Read the model definition and answer for the solid it produces. Units are mm, in the model's axes. A direction names the side the tool comes from. Coordinates: 2 decimals unless noted, no trailing zeros. Write each loop counter-clockwise with the first axis right and the second up, starting at its lowest first coordinate (ties: lowest second). Pieces come first, ordered by that corner, then holes. Notation, with made-up numbers: (-35.75, -10) -> (0.25, -10) arc R30 cw to (0.25, 19) -> close; hole circle Ø11 at (1, 86.25). An arc over 180 degrees is marked (long way). Write item = value, one per line. Start each with the question number.
1) Flat-ended cylindrical pins translate along their axes: pin 1 Ø5 at (x, z) = (10, 192.75) entering from +Y; pin 2 Ø5 at (y, z) = (10, 207) entering from +X. Find the tip coordinate at first contact, or state that the pin passes through.
2) A tool of negligible diameter and unlimited length cuts with its end or side. For faces 1 (the face through (4, 6, 0)), 2 (the face through (10, 5, 173)), from which of +Z, -Z, +X, -X, +Y, -Y can it reach the whole face along a straight path? Write none if from no direction.
3) Section A-A (y = 2.75) is taken. Count the separate pieces of the cut face and the enclosed holes in it, plus the area to 3 significant figures.
4) Find the intervals of material crossed by line 1 along X through (y, z) = (2.5, 342.55); line 2 along X through (y, z) = (12.25, 227), in increasing order. Write a range as from..to.
5) Section B-B (z = 247.5) is taken. Determine the outline of the cut face in (x, y), plus the area to 3 significant figures.
from build123d import *

# Parameters (mm, degrees)
BOSS_EXTRUDE1_DEPTH                  = 350
F_3_2_3_2_DIAMETER_HOLE1_D           = 3.2
LPATTERN2_COUNT                      = 4
LPATTERN2_PITCH                      = 74.9
F_3_2_3_2_DIAMETERHOLEFORAHALFPART_D = 3.2


with BuildPart() as part:
    # Sketch1 → Boss-Extrude1 (new body)
    with BuildSketch(Plane.XY):
        Polygon((0, 0), (0, 15), (5, 15), (5, 5), (15, 5), (15, 0), align=None)
    extrude(amount=BOSS_EXTRUDE1_DEPTH)

    # Ø3.2 (3.2) Diameter Hole1 (through all)
    with Locations(Plane(origin=(0, 0, 0), x_dir=(-1, 0, 0), z_dir=(0, -1, 0))):
        with Locations((-10, -342.55), (-10, -282.55)):
            f_3_2_3_2_diameter_hole1 = Hole(F_3_2_3_2_DIAMETER_HOLE1_D / 2)

    # LPattern2: Ø3.2 (3.2) Diameter Hole1 ×4
    with Locations(*[(0, 0, -i * LPATTERN2_PITCH) for i in range(1, LPATTERN2_COUNT)]):
        add(f_3_2_3_2_diameter_hole1, mode=Mode.SUBTRACT)

    # Ø3.2 (3.2) DiameterHoleForAHalfPart (through all)
    with Locations(Plane(origin=(0, 0, 0), x_dir=(-1, 0, 0), z_dir=(0, -1, 0))):
        with Locations((-10, -42.95), (-10, -12.95)):
            Hole(F_3_2_3_2_DIAMETERHOLEFORAHALFPART_D / 2)


solid = part.part
Answer key:
q1.pin_1 = 5
q1.pin_2 = 5
q2.face_1 = -Z, +X, -X, +Y, -Y
q2.face_2 = +Z, -Z, +X, +Y
q3.separate_pieces = 1
q3.enclosed_holes = 10
q3.area = 5,170 mm^2
q4.line_1 = 0..8.4, 11.6..15
q4.line_2 = 0..5
q5.outline = (0, 0) -> (15, 0) -> (15, 5) -> (5, 5) -> (5, 15) -> (0, 15) -> close
q5.area = 125 mm^2
